Study the drawing (mm; zero at the part's minimum x, y, z) and answer. Round coordinates to 2 decimals unless told otherwise and drop trailing zeros. Write each loop counter-clockwise with the first axis right and the second up, starting at its lowest first coordinate (ties: lowest second). Pieces come first, ordered by that corner, then holes. Notation, with made-up numbers: M -23.5,79 L 4.5,79 A12 ccw 4.5,95 Z; hole C -20,62 d5. An arc over 180 degrees is marked long. Put each result on its own line as item: value. Start each with the question number.
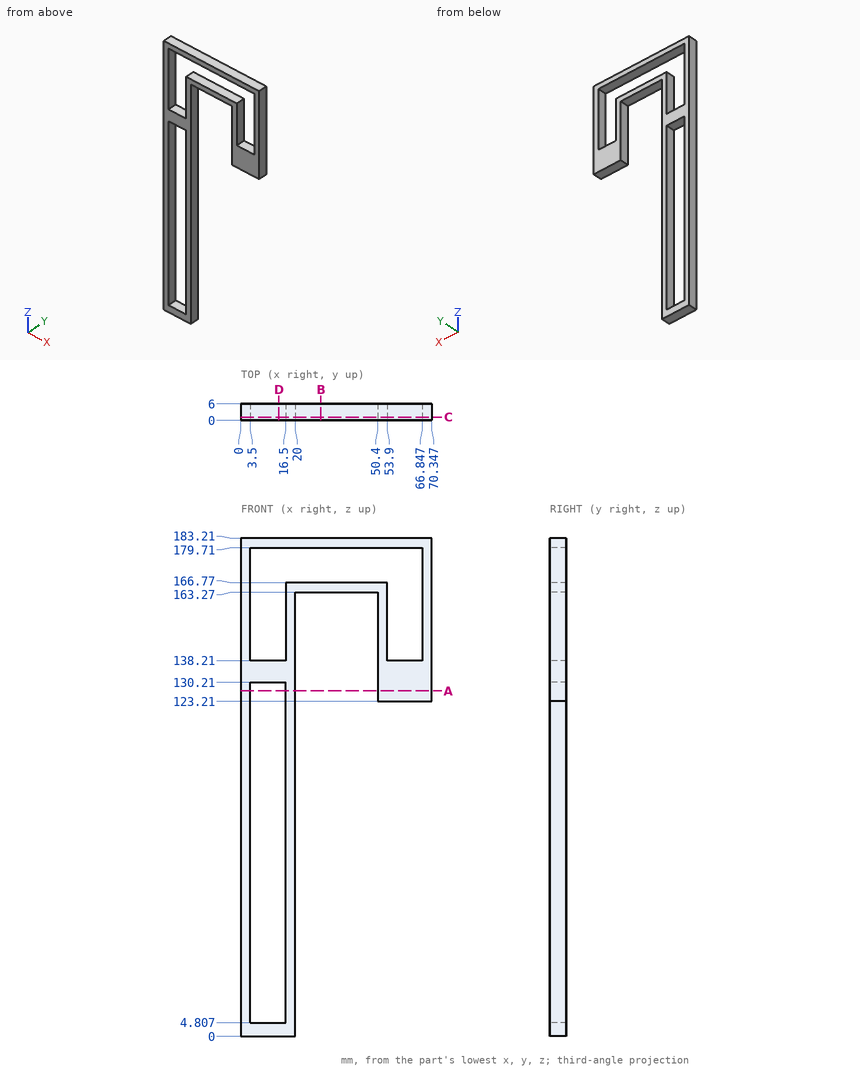
Item 1: Section A-A (z = 127) is taken. Give the vertices of the cut face in (x, y), and give its area (3 significant figures).
Item 2: Flat-ended cylindrical pins translate along their axes: pin 1 (1.8 mm diameter, centred on x = 56.5, y = 4, fed in from -Z); pin 2 (3 mm diameter, centred on x = 24.5, y = 1.5, fed in from -Z). Find the tip coordinate at first contact, or state that the pin passes through.
Item 3: Consider line 1 along Z through (x, y) = (7, 3.05); line 2 along X through (y, z) = (0.65, 129.5); line 3 along Z through (x, y) = (21, 2.65). Determine where each line is inside the solid, lowest interval first. Write a range as [from, to].
Item 4: Section D-D (x = 14) is taken. Give the vertices of the cut face in (y, z).
Item 5: Section B-B (x = 29.5) is taken. Give the vertices of the cut face in (y, z).
Item 6: Section C-C (y = 1.2) is taken. Give the vertices of the cut face in (x, z), and give its area (3 significant figures).
Output values:
1. outline: M 0,0 L 3.5,0 L 3.5,6 L 0,6 Z; M 16.5,0 L 20,0 L 20,6 L 16.5,6 Z; M 50.4,0 L 70.35,0 L 70.35,6 L 50.4,6 Z
1. area: 162 mm^2
2. pin 1: stops at z = 123.21
2. pin 2: stops at z = 163.27
3. line 1: z = [0, 4.81], [130.21, 138.21], [179.71, 183.21]
3. line 2: x = [0, 3.5], [16.5, 20], [50.4, 70.35]
3. line 3: z = [163.27, 166.77], [179.71, 183.21]
4. outline: M 0,0 L 6,0 L 6,4.81 L 0,4.81 Z; M 0,130.21 L 6,130.21 L 6,138.21 L 0,138.21 Z; M 0,179.71 L 6,179.71 L 6,183.21 L 0,183.21 Z
5. outline: M 0,163.27 L 6,163.27 L 6,166.77 L 0,166.77 Z; M 0,179.71 L 6,179.71 L 6,183.21 L 0,183.21 Z
6. outline: M 0,0 L 20,0 L 20,163.27 L 50.4,163.27 L 50.4,123.21 L 70.35,123.21 L 70.35,183.21 L 0,183.21 Z; hole M 3.5,4.81 L 16.5,4.81 L 16.5,130.21 L 3.5,130.21 Z; hole M 3.5,138.21 L 16.5,138.21 L 16.5,166.77 L 53.9,166.77 L 53.9,138.21 L 66.85,138.21 L 66.85,179.71 L 3.5,179.71 Z
6. area: 2,280 mm^2
